Geometry check sheet. Reference: the model listing, model coordinates, mm. A direction names the side the tool comes from. Round coordinates to 2 decimals unless told otherwise and drop trailing zeros. Order: outer loops, then holes, each group sorted by start corner. A loop starts at its lowest first (then second) coordinate and runs counter-clockwise, first axis right, second up. Notation, with made-up numbers: (82.5, 62.5) -> (108.5, 62.5) arc R16 cw to (108.5, 75.5) -> close; hole circle Ø1 at (13, -8.5). An arc over 180 degrees is marked (long way). Answer as a JSON object with one key per item and string values. Group by question number.
from build123d import *

# Parameters (mm, degrees)
BOSS_EXTRUDE1_DEPTH      = 2
BOSS_EXTRUDE1_DEPTH_BACK = 1
SKETCH3_W                = 47.4
SKETCH3_H                = 42.1
SKETCH4_W                = 2.2
SKETCH4_H                = 5
BOSS_EXTRUDE2_DEPTH      = 9
SKETCH6_W                = 2.2
SKETCH6_H                = 3
BOSS_EXTRUDE3_DEPTH      = 9.8
BOSS_EXTRUDE5_REACH      = 57.819
SKETCH10_W               = 9.8
SKETCH10_H               = 3
MIRROR3_COPY_1_SKETCH_W  = 2.2
MIRROR3_COPY_1_SKETCH_H  = 5
MIRROR3_COPY_1_DEPTH     = 9
MIRROR3_COPY_2_SKETCH_W  = 2.2
MIRROR3_COPY_2_SKETCH_H  = 3
MIRROR3_COPY_2_DEPTH     = 9.8
SKETCH7_W                = 8
SKETCH7_H                = 8
CUT_EXTRUDE1_DEPTH       = 3
SKETCH12_W               = 47.4
SKETCH12_H               = 42.1
BOSS_EXTRUDE6_DEPTH      = 6


with BuildPart() as part:
    # Sketch3 → Boss-Extrude1 (new, two sides: drawn at the far end of the back side and taken through both)
    with BuildSketch(Plane(origin=(0, 0, 0), x_dir=(1, 0, 0), z_dir=(0, 1, 0)).offset(-BOSS_EXTRUDE1_DEPTH_BACK)):
        Rectangle(SKETCH3_W, SKETCH3_H)
    extrude(amount=BOSS_EXTRUDE1_DEPTH + BOSS_EXTRUDE1_DEPTH_BACK)

    # Sketch4 → Boss-Extrude2 (add)
    with BuildSketch(Plane(origin=(0, 2, 0), x_dir=(1, 0, 0), z_dir=(0, 1, 0))):
        with Locations((-22.6, 18.55)):
            Rectangle(SKETCH4_W, SKETCH4_H)
    boss_extrude2 = extrude(amount=BOSS_EXTRUDE2_DEPTH)

    # Sketch6 → Boss-Extrude3 (add)
    with BuildSketch(Plane(origin=(0, 0, -21.05), x_dir=(-1, 0, 0), z_dir=(0, 0, -1))):
        with Locations((22.6, 9.5)):
            Rectangle(SKETCH6_W, SKETCH6_H)
    boss_extrude3 = extrude(amount=BOSS_EXTRUDE3_DEPTH)

    # Mirror1: Boss-Extrude2, Boss-Extrude3 across plane
    add(boss_extrude2.mirror(Plane(origin=(0, 0, 0), x_dir=(0, 0, 1), z_dir=(1, 0, 0))))
    add(boss_extrude3.mirror(Plane(origin=(0, 0, 0), x_dir=(0, 0, 1), z_dir=(1, 0, 0))))

    # Sketch10 → Boss-Extrude5 (add, up to next)
    with BuildSketch(Plane(origin=(-21.5, 0, 0), x_dir=(0, 0, -1), z_dir=(1, 0, 0)), mode=Mode.PRIVATE) as boss_extrude5_sk1:
        with Locations((25.95, 9.5)):
            Rectangle(SKETCH10_W, SKETCH10_H)
    boss_extrude5_tool1 = extrude(boss_extrude5_sk1.sketch, amount=BOSS_EXTRUDE5_REACH, mode=Mode.PRIVATE) - part.part
    boss_extrude5 = boss_extrude5_tool1.solids().sort_by_distance((-21.5, 9.5, -25.95))[0]
    add(boss_extrude5)

    # Mirror3: Boss-Extrude2, Boss-Extrude3, Boss-Extrude5 across plane
    add(boss_extrude2.mirror(Plane.XY))
    add(boss_extrude3.mirror(Plane.XY))
    add(boss_extrude5.mirror(Plane.XY))

    # Mirror3 copy 1 sketch → Mirror3 copy 1 (add)
    with BuildSketch(Plane(origin=(0, 2, 0), x_dir=(-1, 0, 0), z_dir=(0, 1, 0))):
        with Locations((-22.6, 18.55)):
            Rectangle(MIRROR3_COPY_1_SKETCH_W, MIRROR3_COPY_1_SKETCH_H)
    extrude(amount=MIRROR3_COPY_1_DEPTH)

    # Mirror3 copy 2 sketch → Mirror3 copy 2 (add)
    with BuildSketch(Plane.XY.offset(21.05)):
        with Locations((22.6, 9.5)):
            Rectangle(MIRROR3_COPY_2_SKETCH_W, MIRROR3_COPY_2_SKETCH_H)
    extrude(amount=MIRROR3_COPY_2_DEPTH)

    # Sketch7 → Cut-Extrude1 (cut)
    with BuildSketch(Plane.XZ.offset(1)):
        Rectangle(SKETCH7_W, SKETCH7_H)
    extrude(amount=-CUT_EXTRUDE1_DEPTH, mode=Mode.SUBTRACT)

    # Sketch12 → Boss-Extrude6 (add)
    with BuildSketch(Plane.XZ.offset(1)):
        Rectangle(SKETCH12_W, SKETCH12_H)
    extrude(amount=BOSS_EXTRUDE6_DEPTH)

    # loft from a face of the part (cut_loft1)
    loft([part.faces().sort_by_distance((0, -7, 0))[0], part.faces().sort_by_distance((0, -1, 0))[0]], mode=Mode.SUBTRACT)


solid = part.part
Item 1: Sectioned sample at D-D, the plane z = 26. Enter the section's corners in (x, y), then the cut area to 3 significant figures.
Item 2: Mould release check, pull along X, two halves, no side actions. Record for faces 1 (the flat face through (0, 9, -21.05)), 2 (the flat face through (-23, 6, -16.05)): pulls with the +X half, pulls with the -X half, needs draft (parallel to the pull), parting line crosses it, or undercut.
Item 3: Sectioned sample at B-B, the plane y = 0.25. Enter the section's corners in (x, z), then the cut area to 3 significant figures.
Item 4: Thickness scan on L1, parallel to X at y = 9.25, z = 17.5; L2, parallel to Z at x = 5, y = 0.5; L3, parallel to Y at x = 9, z = 22.5. Record the ranges inside material, lowest first.
Item 5: Depth check by flat-ended pin: pin 1 Ø4 at (x, z) = (2.5, -15.5) entering from +Y; pin 2 Ø4.5 at (x, y) = (-10.5, -1) entering from +Z; pin 3 Ø1 at (x, z) = (12.5, 8) entering from -Y. Enter the tip coordinate at first touch or a pass-through.
Item 6: Sectioned sample at C-C, the plane x = 2. Count the separate pieces of the cut face and the enclosed holes in it, then the cut area to 3 significant figures.
Item 7: Sectioned sample at A-A, the plane y = 9. Enter the section's corners in (x, z), then the cut area to 3 significant figures.
Item 8: Set-up check for faces 3 (the flat face through (4, 0, 0)), 4 (the flat face through (0, -3, 21.05)), 5 (the flat face through (-23, 6, 16.05)), 6 (the flat face through (21.5, 6, -19)): record each of +Z, -Z, +X, -X, +Y, -Y from which the full face is reachable in a straight line by a thin tool's end or side.
Result:
{
 "1": {"outline": "(-23.7, 8) -> (23.7, 8) -> (23.7, 11) -> (-23.7, 11) -> close", "area": "142 mm2"},
 "2": {"face 1": "undercut", "face 2": "needs draft"},
 "3": {"outline": "(-23.7, -21.05) -> (23.7, -21.05) -> (23.7, 21.05) -> (-23.7, 21.05) -> close; hole (-4, -4) -> (4, -4) -> (4, 4) -> (-4, 4) -> close", "area": "1,930 mm2"},
 "4": {"L1": "x = -23.7 to -21.5, 21.5 to 23.7", "L2": "z = -21.05 to 21.05", "L3": "y = 8 to 11"},
 "5": {"pin 1": "stops at y = 2", "pin 2": "stops at z = 21.05", "pin 3": "stops at y = -3.74"},
 "6": {"separate pieces": "4", "enclosed holes": "0", "area": "263 mm2"},
 "7": {"outline": "(-23.7, -30.85) -> (23.7, -30.85) -> (23.7, -16.05) -> (21.5, -16.05) -> (21.5, -21.05) -> (-21.5, -21.05) -> (-21.5, -16.05) -> (-23.7, -16.05) -> close; (-23.7, 16.05) -> (-21.5, 16.05) -> (-21.5, 21.05) -> (21.5, 21.05) -> (21.5, 16.05) -> (23.7, 16.05) -> (23.7, 30.85) -> (-23.7, 30.85) -> close", "area": "973 mm2"},
 "8": {"face 3": "+Y, -Y", "face 4": "+Z, +X, -X, -Y", "face 5": "+X, -X, +Y", "face 6": "+Y"}
}
